Read the model definition and answer for the solid it produces. Units are mm, in the model's axes. Give positions to 0.01 mm unless a question says otherwise; leave off trailing zeros. Loops run counter-clockwise (first coordinate to the right, second up) from the corner with the lowest first, then second, coordinate; pieces in that order, holes last. Notation, with made-up numbers: (-26, 63.25) - (33, 63.25) arc R27 cw to (33, 94.25) - close; hole circle Ø1 at (7, 52.25). An arc over 180 degrees is marked (long way). Use a Markdown table: item, result. Add a question column.
Item 1: A cutting plane is placed at A-A (y = 0.4). Determine the outline of the cut face in (x, z).
Item 2: A cutting plane is placed at B-B (x = -1.25). Determine the outline of the cut face in (y, z).
Item 3: For a pull along X with two mould halves and no side action, classify faces 1 (the face through (-3.5, 1, 0)), 2 (the face through (0, 1, -2.51)), 3 (the face through (2.68, 0.64, 2.31)) as +X half, -X half, draft (parallel to the pull), parting line (faces both ways), or undercut.
Item 4: Consider probe 1 along Z at (x, y) = (-2.25, 1.4); probe 2 along Y at (x, z) = (3.25, -0.6); probe 3 along X at (y, z) = (1.75, 1.6). Determine where each line is inside the solid, lowest interval first. Write a range as [from, to].
Item 5: A cutting plane is placed at C-C (z = -0.5). Determine the outline of the cut face in (x, y), plus the area to 4 significant figures.
from build123d import *

# Parameters (mm, degrees)
EXTRUDE_1_DEPTH = 1.8
CHAMFER_1_SIZE  = 0.5


with BuildPart() as part:
    # Эскиз1 → Бобышка-Вытянуть1 (new body)
    with BuildSketch(Plane(origin=(0, 0, 0), x_dir=(1, 0, 0), z_dir=(0, 1, 0))):
        with BuildLine():
            Line((-3.5, 2.51), (-3.210140252, 2.51))
            ThreePointArc((-3.210140252, 2.51), (-2.673786949, 2.310468426), (-2.137433645, 2.51))
            Line((-2.137433645, 2.51), (2.137433645, 2.51))
            ThreePointArc((2.137433645, 2.51), (2.673786949, 2.310468426), (3.210140252, 2.51))
            Line((3.210140252, 2.51), (3.5, 2.51))
            Line((3.5, 2.51), (3.5, -2.51))
            Line((3.5, -2.51), (3.210140252, -2.51))
            ThreePointArc((3.210140252, -2.51), (2.673786949, -2.310468426), (2.137433645, -2.51))
            Line((2.137433645, -2.51), (-2.137433645, -2.51))
            ThreePointArc((-2.137433645, -2.51), (-2.673786949, -2.310468426), (-3.210140252, -2.51))
            Line((-3.210140252, -2.51), (-3.5, -2.51))
            Line((-3.5, -2.51), (-3.5, 2.51))
        make_face()
    extrude(amount=EXTRUDE_1_DEPTH)

    # Фаска1
    chamfer_1_edges = [part.edges().sort_by_distance(p)[0] for p in [
        (-3.5, 1.8, 0),
    ]]
    chamfer(chamfer_1_edges, length=CHAMFER_1_SIZE)
    chamfer_1_2_edges = [part.edges().sort_by_distance(p)[0] for p in [
        (3.5, 1.8, 0),
    ]]
    chamfer(chamfer_1_2_edges, length=CHAMFER_1_SIZE)
    chamfer_1_3_edges = [part.edges().sort_by_distance(p)[0] for p in [
        (-2.54973161, 1.8, 2.319899262),
    ]]
    chamfer(chamfer_1_3_edges, length=CHAMFER_1_SIZE)
    chamfer_1_4_edges = [part.edges().sort_by_distance(p)[0] for p in [
        (-2.54973161, 1.8, -2.319899262),
    ]]
    chamfer(chamfer_1_4_edges, length=CHAMFER_1_SIZE)
    chamfer_1_5_edges = [part.edges().sort_by_distance(p)[0] for p in [
        (2.54973161, 1.8, -2.319899262),
    ]]
    chamfer(chamfer_1_5_edges, length=CHAMFER_1_SIZE)
    chamfer_1_6_edges = [part.edges().sort_by_distance(p)[0] for p in [
        (2.54973161, 1.8, 2.319899262),
    ]]
    chamfer(chamfer_1_6_edges, length=CHAMFER_1_SIZE)
    chamfer_1_7_edges = [part.edges().sort_by_distance(p)[0] for p in [
        (0, 1.8, -2.51),
    ]]
    chamfer(chamfer_1_7_edges, length=CHAMFER_1_SIZE)
    chamfer_1_8_edges = [part.edges().sort_by_distance(p)[0] for p in [
        (0, 1.8, 2.51),
    ]]
    chamfer(chamfer_1_8_edges, length=CHAMFER_1_SIZE)


solid = part.part
Geometry says:
| question | item | result |
|---|---|---|
| 1 | outline | (-3.5, -2.51) - (-3.21, -2.51) arc R0.82 cw to (-2.14, -2.51) - (2.14, -2.51) arc R0.82 cw to (3.21, -2.51) - (3.5, -2.51) - (3.5, 2.51) - (3.21, 2.51) arc R0.82 cw to (2.14, 2.51) - (-2.14, 2.51) arc R0.82 cw to (-3.21, 2.51) - (-3.5, 2.51) - close |
| 2 | outline | (0, -2.51) - (1.3, -2.51) - (1.8, -2.01) - (1.8, 2.01) - (1.3, 2.51) - (0, 2.51) - close |
| 3 | face 1 | -X half |
| 3 | face 2 | draft |
| 3 | face 3 | undercut |
| 4 | probe 1 | [-2.31, 2.31] |
| 4 | probe 2 | [0, 1.55] |
| 4 | probe 3 | [-3.05, 3.05] |
| 5 | outline | (-3.5, 0) - (3.5, 0) - (3.5, 1.3) - (3, 1.8) - (-3, 1.8) - (-3.5, 1.3) - close |
| 5 | area | 12.35 mm² |
